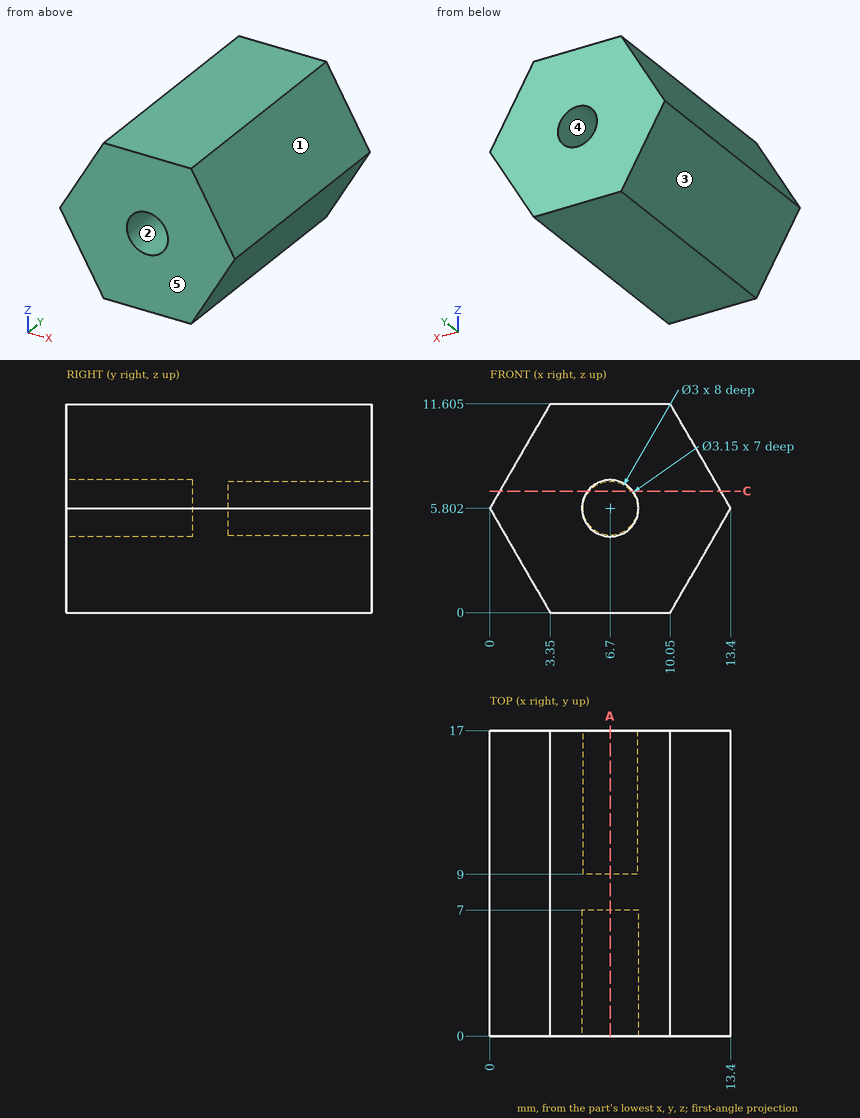
Could you check a few things on this drawing? It's one solid part, dimensions in mm from its lowest x, y, z. A direction names the side the tool comes from. Round coordinates to 2 decimals unless told otherwise and drop trailing zeros. Write each loop counter-clockwise with the first axis right and the second up, starting at its lowest first coordinate (ties: lowest second). Pieces come first, ordered by that corner, then holes. Notation, with made-up numbers: (58.25, 42.5) -> (64.25, 42.5) arc R22 ccw to (64.25, 56.5) -> close; hole circle Ø8 at (-31, 81). An arc over 180 degrees is marked (long way). One line per question, with ' | ' between items. Start each with the question number.
1) If we mould it in two halves opening along Z, with no side actions, what happens to the marked faces 1, 2 and 3? For each: released by +Z, released by -Z, zero draft, split by the parting line, or undercut.
2) On a 3-axis mill with a long thin cutter (end or side, diameter ignored), from which of +Z, -Z, +X, -X, +Y, -Y can I reach the whole of each face in a straight line? I mean the marked faces 4 and 5. Say none if no direction works.
3) Suppose I cut it at A-A on x = 6.7. Write out the boundary of the cut face in (y, z) (1 decimal), then the cut area to 3 significant figures.
4) I'm going to push flat-ended pins straight in: P1, Ø2.5, axis at x = 6.7, z = 5.8, coming from the -Y side; P2, Ø5, axis at y = 3.5, z = 7.5, coming from the -X side; P3, Ø1.5, axis at x = 6.5, z = 6, coming from the +Y side. Where does each tip first touch, or does it pass through?
5) I need wall thicknesses on line 1 (Z direction, x = 6.75, y = 2.5) (1 decimal); line 2 (Z direction, x = 6.7, y = 15.25) (1 decimal); line 3 (X direction, y = 15, z = 6.5). Which ranges of each line are inside material? Lowest first, please. Write a range as [from, to].
6) Suppose I cut it at C-C on z = 6.75. Write out the boundary of the cut face in (x, y), then the cut area to 3 significant figures.
Return value:
1) face 1: released by +Z | face 2: undercut | face 3: released by -Z
2) face 4: +Y | face 5: +Z, -Z, +X, -X, -Y
3) outline: (0, 0) -> (17, 0) -> (17, 4.3) -> (9, 4.3) -> (9, 7.3) -> (17, 7.3) -> (17, 11.6) -> (0, 11.6) -> (0, 7.4) -> (7, 7.4) -> (7, 4.2) -> (0, 4.2) -> close | area: 151 mm2
4) P1: stops at y = 7 | P2: stops at x = 0 | P3: stops at y = 9
5) line 1: z = [0, 4.2], [7.4, 11.6] | line 2: z = [0, 4.3], [7.3, 11.6] | line 3: x = [0.4, 5.37], [8.03, 13]
6) outline: (0.55, 0) -> (5.44, 0) -> (5.44, 7) -> (7.96, 7) -> (7.96, 0) -> (12.85, 0) -> (12.85, 17) -> (7.86, 17) -> (7.86, 9) -> (5.54, 9) -> (5.54, 17) -> (0.55, 17) -> close | area: 173 mm2
